Here's how the part is built. I have some questions about the finished solid (model axes, mm). Coordinates: 2 decimals unless noted, no trailing zeros. Loops run counter-clockwise (first coordinate to the right, second up) from the corner with the lowest first, then second, coordinate; pieces in that order, holes last.
Autodesk Inventor part; units mm, degrees
ref_plane "YZ Plane" through (0, 0, 0) normal (1, 0, 0) x (0, 1, 0)
ref_plane "XZ Plane" through (0, 0, 0) normal (0, 1, 0) x (-1, 0, 0)
ref_plane "XY Plane" through (0, 0, 0) normal (0, 0, 1) x (1, 0, 0)
sketch "草圖1" plane through (0, 0, 0) normal (0, 1, 0) x (-1, 0, 0)
  line L0 (-14, 14) -> (14, 14)
  line L1 (14, 14) -> (14, -14)
  line L2 (14, -14) -> (-14, -14)
  line L3 (-14, -14) -> (-14, 14)
  line L4 (-14, 14) -> (14, -14) construction
  line L5 (14, 14) -> (-14, -14) construction
  point P0 (0, 0)
  dimension "d0" = 28
  dimension "d1" = 28
extrude "擠出1" add sketch "草圖1" along normal blind 1.6
sketch "草圖2" plane through (0, 0, 0) normal (1, 0, 0) x (0, 1, 0)
  line L0 (1.6, 14) -> (1.6, -14)
  circle A0 centre (1.6, 0) radius 11.175
  line L1 (12.775, 0) -> (1.6, 0)
  line L2 (-14.045, 0) -> (17.245, 0)
  point P0 (0, 0)
  point P1 (1.6, -11.175)
  dimension "d4" = 22.35
revolve "迴轉1" add sketch "草圖2" angle 360 about axis through (0, -10, 0) along (0, 1, 0) picked at (4.0451, -6.9877) contours L1 A0 L0
sketch "草圖3" plane through (0, 1.6, 0) normal (0, 1, 0) x (1, 0, 0)
  circle A0 centre (0, 0) radius 11.175
  line L0 (14, 14) -> (-14, 14)
  line L1 (-14, 14) -> (-14, -14)
  line L2 (-14, -14) -> (14, -14)
  line L3 (14, -14) -> (14, 14)
  line L4 (11.175, -11.175) -> (-11.175, -11.175) construction
  line L5 (-11.175, -11.175) -> (-11.175, 11.175) construction
  line L6 (-11.175, 11.175) -> (11.175, 11.175) construction
  line L7 (11.175, 11.175) -> (11.175, -11.175) construction
  line L8 (11.175, -11.175) -> (-11.175, 11.175) construction
  line L9 (-11.175, -11.175) -> (11.175, 11.175) construction
  circle A1 centre (-11.175, 11.175) radius 1.5
  circle A2 centre (11.175, -11.175) radius 1.5
  dimension "d6" = 3
  dimension "d7" = 3
extrude "擠出2" cut sketch "草圖3" against normal blind 1.6 contours A1 | A2
properties part number "50w led"
1. I want a section at B-B (z = 12). Please give me the cut outline in (x, y), then the cut area to 3 significant figures.
2. I need wall thicknesses on line 1 along Y through (x, z) = (-1.5, -12.5); line 2 along X through (y, z) = (1, 12); line 3 along Z through (x, y) = (-11.5, 0.5). Which ranges of each line are inside material? Lowest first, please.
3. For pin 1 (1.5 mm diameter, centred on y = 11, z = 3, fed in from +X); pin 2 (3 mm diameter, centred on y = 5, z = 9, fed in from -X); pin 3 (3.5 mm diameter, centred on x = 11.175, z = 11.175, fed in from +Y); pin 4 (1 mm diameter, centred on y = 10, z = -8.5, fed in from +X), each with a flat end and sliding along its axis, tell me the tip position at first contact or that it passes through.
4. I want a section at A-A (y = 1.25). Please give me the cut outline in (x, z) (3 decimals).
5. I want a section at D-D (z = -3.75). Please give me the cut outline in (x, y), then the cut area to 3 significant figures.
6. I want a section at C-C (x = -10.5). Please give me the cut outline in (y, z) (3 decimals).
7. We'd pull the mould along Z, two halves only. Please class faces 1 (the flat face through (0, 1, -14)), 2 (the flat face through (6, 1.6, 10)), 3 (the cylindrical face through (-11.5, 0.81, -9.71)), 4 (the cylindrical face through (12.56, 0.81, 11.75)): +Z half, -Z half, draft (parallel to the pull), parting line (faces both ways), or undercut.
Response values:
1. outline: (-14, 0) - (9.92, 0) - (9.92, 1.6) - (-14, 1.6) - close; (12.43, 0) - (14, 0) - (14, 1.6) - (12.43, 1.6) - close
1. area: 40.8 mm2
2. line 1: y = 0 to 1.6
2. line 2: x = -14 to 9.92, 12.43 to 14
2. line 3: z = -14 to -12.64, -9.71 to 14
3. pin 1: stops at x = 6.46
3. pin 2: stops at x = -7.68
3. pin 3: stops at y = 1.6
3. pin 4: passes through
4. outline: (-14, -14) - (14, -14) - (14, 14) - (-14, 14) - close; hole circle Ø3 at (-11.175, -11.175); hole circle Ø3 at (11.175, 11.175)
5. outline: (-14, 0) - (14, 0) - (14, 1.6) - (10.53, 1.6) arc R10.53 ccw to (-10.53, 1.6) - (-14, 1.6) - close
5. area: 219 mm2
6. outline: (0, -14) - (1.6, -14) - (1.6, -12.515) - (0, -12.515) - close; (0, -9.835) - (1.6, -9.835) - (1.6, -3.825) arc R3.825 ccw to (1.6, 3.825) - (1.6, 14) - (0, 14) - close
7. face 1: -Z half
7. face 2: draft
7. face 3: undercut
7. face 4: undercut
